Can you work these out from the model? Positions are in its coordinate system, mm. A direction names the side the tool comes from. Give positions to 0.01 mm unless a question says otherwise; leave off trailing zeros. Write each loop counter-clockwise with the first axis right and the second up, starting at its lowest first coordinate (ties: lowest second). Pieces come first, ordered by that corner, then holes.
from build123d import *

# Parameters (mm, degrees)
BOSS_EXTRU_1_DEPTH      = 10
ESQUISSE6_R             = 2.05
ESQUISSE6_W             = 10
ESQUISSE6_H             = 21
BOSS_EXTRU_3_DEPTH      = 5
ESQUISSE4_R             = 2.05
ENL_V_MAT_EXTRU_2_DEPTH = 123.869849841
CONG_1_R                = 1.5
ESQUISSE8_R             = 2.05
ENL_V_MAT_EXTRU_4_DEPTH = 15


# Read off the part's stored shape, not the designer's step: Symétrie9
with BuildPart() as part:
    # Esquisse2 → Boss.-Extru.1 (new body)
    with BuildSketch(Plane.XY):
        Polygon((0, 0), (0, 16), (15, 16), (15, 21), (65, 21), (65, 16), (95, 16), (95, 21), (115, 21), (115, 0), align=None)
    extrude(amount=BOSS_EXTRU_1_DEPTH)

    # Esquisse6 → Boss.-Extru.3 (add)
    # profile 1 of 2: a face of its own
    with BuildSketch(Plane(origin=(115, 0, 0), x_dir=(0, 0, -1), z_dir=(1, 0, 0))):
        with BuildLine():
            Line((15.562445841, 0), (18.53122292, 2.96877708))
            ThreePointArc((18.53122292, 2.96877708), (21, 8.928932188), (18.53122292, 14.889087297))
            Line((18.53122292, 14.889087297), (4.389087297, 29.03122292))
            ThreePointArc((4.389087297, 29.03122292), (-4.796680513, 30.858385741), (-10, 23.071067812))
            Line((-10, 23.071067812), (-10, 21))
            Line((-10, 21), (0, 21))
            Line((0, 21), (0, 0))
            Line((0, 0), (15.562445841, 0))
        make_face()
        with Locations(Location((12.571067812, 8.928932188, 0), (0, 0, 90))):
            Circle(ESQUISSE6_R, mode=Mode.SUBTRACT)
        with Locations(Location((-1.571067812, 23.071067812, 0), (0, 0, 90))):
            Circle(ESQUISSE6_R, mode=Mode.SUBTRACT)
    # profile 2 of 2: a face of its own
    with BuildSketch(Plane(origin=(115, 0, 0), x_dir=(0, 0, -1), z_dir=(1, 0, 0))):
        with Locations((-5, 10.5)):
            Rectangle(ESQUISSE6_W, ESQUISSE6_H)
    extrude(amount=BOSS_EXTRU_3_DEPTH)

    # Esquisse4 → Enlèv. mat.-Extru.2 (cut, symmetric)
    with BuildSketch(Plane(origin=(0, 16, 0), x_dir=(1, 0, 0), z_dir=(0, 1, 0))):
        with Locations(Location((8, -5, 0), (0, 0, 180))):
            Circle(ESQUISSE4_R)
        with Locations(Location((72, -5, 0), (0, 0, 180))):
            Circle(ESQUISSE4_R)
        with Locations((88, -5)):
            Circle(ESQUISSE4_R)
    extrude(amount=ENL_V_MAT_EXTRU_2_DEPTH, both=True, mode=Mode.SUBTRACT)

    # Congé1
    cong_1_edges = [part.edges().sort_by_distance(p)[0] for p in [
        (40, 21, 0),
        (105, 21, 10),
        (105, 21, 0),
        (40, 21, 10),
        (115, 21.960155108, -11.460155108),
        (115, 8.928932188, -21),
        (115, 1.48438854, -17.04683438),
        (115, 22.035533906, 10),
        (120, 1.48438854, -17.04683438),
        (120, 8.928932188, -21),
        (120, 21.960155108, -11.460155108),
        (115, 30.858385741, 4.796680513),
        (120, 11.535533906, 10),
        (120, 30.858385741, 4.796680513),
    ]]
    fillet(cong_1_edges, radius=CONG_1_R)

    # Esquisse8 → Enlèv. mat.-Extru.4 (cut)
    # profile 1 of 2: a face of its own
    with BuildSketch(Plane.ZY.offset(-115)):
        with BuildLine():
            ThreePointArc((0, 19.5), (0.439339828, 20.560660172), (1.5, 21))
            Line((1.5, 21), (5.566149553, 21))
            ThreePointArc((5.566149553, 21), (5.943016338, 22.005203804), (6.071067812, 23.071067812))
            ThreePointArc((6.071067812, 23.071067812), (-0.996050694, 26.766998355), (0, 18.85422706))
            Line((0, 18.85422706), (0, 19.5))
        make_face()
        with Locations(Location((1.571067812, 23.071067812, 0), (0, 0, 90))):
            Circle(ESQUISSE8_R, mode=Mode.SUBTRACT)
    # profile 2 of 2: a face of its own
    with BuildSketch(Plane.ZY.offset(-115)):
        with BuildLine():
            Line((5.566149553, 21), (1.5, 21))
            ThreePointArc((1.5, 21), (0.439339828, 20.560660172), (0, 19.5))
            Line((0, 19.5), (0, 18.85422706))
            ThreePointArc((0, 18.85422706), (3.189723507, 18.872263966), (5.566149553, 21))
        make_face()
    extrude(amount=ENL_V_MAT_EXTRU_4_DEPTH, mode=Mode.SUBTRACT)

    # Symétrie9: part across plane


with BuildPart() as part_1:
    add(part.part)
    add(part.part.mirror(Plane(origin=(0, 0, 10), x_dir=(0, 0, 1), z_dir=(1, 0, 0))))


solid = part_1.part
(1) If I drill on L1, parallel to Z at x = 88, y = 4.75; L2, parallel to X at y = 16.5, z = -8.5; L3, parallel to Z at x = 3, y = 12, over which ranges is the centre line in solid material (lowest first)?
Returned:
L1: z = 0 to 2.95, 7.05 to 10
L2: x = -120 to -115, 115 to 120
L3: z = 0 to 10
(2) Imagine slicing it at C-C, the plane x = -106. Write out the boundary of the cut face in (y, z), plus the area to 3 significant figures.
Returned:
outline: (0, 0) - (18.85, 0) arc R4.5 cw to (21, 5.57) - (21, 8.5) arc R1.5 ccw to (19.5, 10) - (0, 10) - close
area: 199 mm2
(3) Will these pins go through, and if not, where does the flat tip stop? P1, Ø3.5, axis at y = 8.93, z = -12.57, coming from the -X side; P2, Ø1, axis at x = -44, y = 16, coming from the -Z side; P3, Ø5.5, axis at y = 23.07, z = 1.57, coming from the +X side; P4, Ø1, axis at x = -49.5, y = 21, coming from the +Z side.
Returned:
P1: passes through
P2: stops at z = 0
P3: stops at x = 120
P4: stops at z = 9.62
(4) Imagine slicing it at B-B, the plane x = 97. Write out the boundary of the cut face in (y, z), plus the area to 3 significant figures.
Returned:
outline: (0, 0) - (19.5, 0) arc R1.5 ccw to (21, 1.5) - (21, 8.5) arc R1.5 ccw to (19.5, 10) - (0, 10) - close
area: 209 mm2
(5) If we mould it in two halves opening along Z, with no side actions, what happens to faces 1 (the face through (107.605, 18.856, 3.147)), 2 (the face through (120, 12, -2)), 3 (the face through (-119.55, 1.73, -16.69))? For each: +Z half, -Z half, draft (parallel to the pull), parting line (faces both ways), or undercut.
Returned:
face 1: undercut
face 2: draft
face 3: -Z half
(6) For faces 4 (the face through (115.428, 21.74, -11.042)), 5 (the face through (-40, 21, 5)), 6 (the face through (10.05, 8.11, 5.09)), 7 (the face through (-115.428, 1.749, -16.673)), which set-ups out of +Z, -Z, +X, -X, +Y, -Y let a thin tool reach every point of the face, with its end or its side?
Returned:
face 4: -Z, +Y
face 5: +Z, -Z, +Y
face 6: +Y, -Y
face 7: -Z, -Y
(7) Imagine slicing it at A-A, the plane x = -72. Write out the boundary of the cut face in (y, z), plus the area to 3 significant figures.
Returned:
outline: (0, 0) - (16, 0) - (16, 2.95) - (0, 2.95) - close; (0, 7.05) - (16, 7.05) - (16, 10) - (0, 10) - close
area: 94.4 mm2
